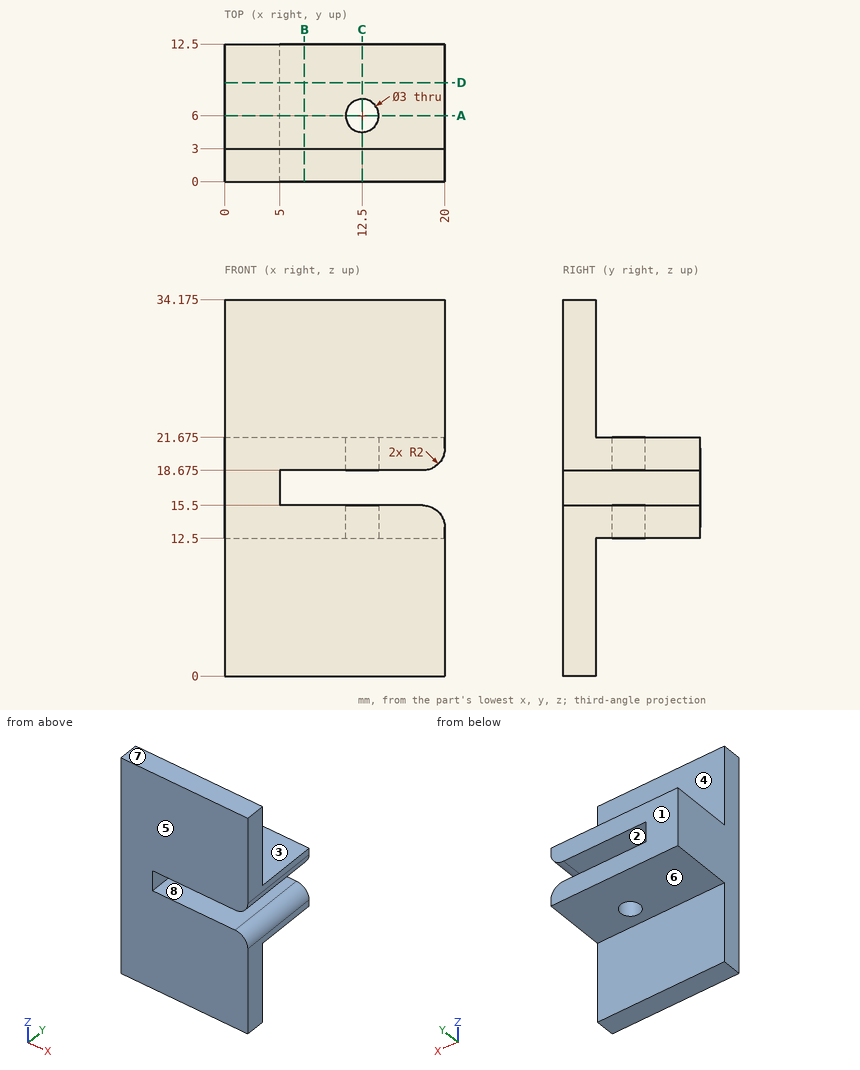
Print and shaded views of the part. All mm, measured from the part's lowest x, y and z. A direction names the side the tool comes from. Coordinates: 2 decimals unless noted, no trailing zeros. Order: outer loops, then holes, each group sorted by start corner. A loop starts at its lowest first (then second) coordinate and runs counter-clockwise, first axis right, second up. Notation, with made-up numbers: M -11.75,-11 L -3.75,-11 A8 cw -3.75,4 Z; hole C 33,35.25 d6. An arc over 180 degrees is marked long. Write each question's results on one line, items separated by ' | '. Start each with the question number.
Q1. Cut at A-A (y = 6). List the corners of the cut face in (x, z) (3 decimals).
Q2. Cut at D-D (y = 9). List the corners of the cut face in (x, z) (3 decimals).
Q3. Drill centre lines: probe 1 along Y at (x, z) = (12.5, 20.8); probe 2 along Z at (x, y) = (14, 10) (3 decimals); probe 3 along Z at (x, y) = (3.5, 7) (3 decimals). Where is each one in solid material? Low to high. Write a range as from..to.
Q4. Which spindle directions (+Z, -Z, +X, -X, +Y, -Y) get a long thin tool onto all of the face, cutting with end or side? Do the marked faces 4, 5, 6, 7 and 8. Say none if no direction does.
Q5. Flat gauge pins, fed straight in: P1, Ø10, axis at x = 9, z = 30.5, coming from the +Y side; P2, Ø3, axis at x = 6.5, y = 6.5, coming from the -Z side; P3, Ø1.6, axis at y = 8.5, z = 17.5, coming from the +X side. Where does each tip first touch, or does it go through?
Q6. Cut at B-B (x = 7.25). List the corners of the cut face in (y, z) (3 decimals), then the cut area to 3 significant figures.
Q7. Pull direction Z, two halves, no side cores. Call the marked faces 1, 2 and 3: +Z half, -Z half, draft (parallel to the pull), parting line (faces both ways), or undercut.
Q8. Cut at C-C (x = 12.5). List the corners of the cut face in (y, z) (3 decimals).
Found:
1) outline: M 0,12.5 L 11,12.5 L 11,15.5 L 5,15.5 L 5,18.675 L 11,18.675 L 11,21.675 L 0,21.675 Z; M 14,12.5 L 20,12.5 L 20,13.5 A2 ccw 18,15.5 L 14,15.5 Z; M 14,18.675 L 18,18.675 A2 ccw 20,20.675 L 20,21.675 L 14,21.675 Z
2) outline: M 0,12.5 L 20,12.5 L 20,13.5 A2 ccw 18,15.5 L 5,15.5 L 5,18.675 L 18,18.675 A2 ccw 20,20.675 L 20,21.675 L 0,21.675 Z
3) probe 1: 0..4.5, 7.5..12.5 | probe 2: 12.5..15.5, 18.675..21.675 | probe 3: 12.5..21.675
4) face 4: +Z, +X, -X, +Y | face 5: +Z, -Z, +X, -X, -Y | face 6: -Z, +X, -X, +Y | face 7: +Z, +X, -X, +Y, -Y | face 8: +X, +Y, -Y
5) P1: y = 3 | P2: z = 12.5 | P3: x = 5
6) outline: M 0,0 L 3,0 L 3,12.5 L 12.5,12.5 L 12.5,15.5 L 0,15.5 Z; M 0,18.675 L 12.5,18.675 L 12.5,21.675 L 3,21.675 L 3,34.175 L 0,34.175 Z | area: 150 mm²
7) face 1: draft | face 2: undercut | face 3: +Z half
8) outline: M 0,0 L 3,0 L 3,12.5 L 4.5,12.5 L 4.5,15.5 L 0,15.5 Z; M 0,18.675 L 4.5,18.675 L 4.5,21.675 L 3,21.675 L 3,34.175 L 0,34.175 Z; M 7.5,12.5 L 12.5,12.5 L 12.5,15.5 L 7.5,15.5 Z; M 7.5,18.675 L 12.5,18.675 L 12.5,21.675 L 7.5,21.675 Z
